```python
from build123d import *

# Parameters (mm, degrees)
BOSS_EXTRUDE1_DEPTH     = 35
SKETCH3_R               = 1.575
CUT_EXTRUDE1_DEPTH      = 10
CUT_EXTRUDE2_DEPTH      = 79.70196948
CUT_EXTRUDE2_DEPTH_BACK = 10
SKETCH5_W               = 10
SKETCH5_H               = 16
FILLET2_R               = 12
FILLET3_R               = 3
FILLET4_R               = 1.5
SKETCH6_W               = 3
SKETCH6_H               = 5.976707935
BOSS_EXTRUDE2_DEPTH     = 15
SKETCH8_R               = 1.125
CUT_EXTRUDE3_DEPTH      = 25
SKETCH10_R              = 3
BOSS_EXTRUDE3_DEPTH     = 3.044394089
SKETCH11_R              = 1.575
CUT_EXTRUDE4_DEPTH      = 7.5


with BuildPart() as part:
    # Sketch2 → Boss-Extrude1 (new body)
    with BuildSketch(Plane.XY):
        Polygon((27, 21), (27, 37), (30, 37), (30, 3), (19, 3), (19, 6), (27, 6), (27, 18), (-27, 18), (-27, 6), (-19, 6), (-19, 3), (-30, 3), (-30, 21), align=None)
    extrude(amount=-BOSS_EXTRUDE1_DEPTH)

    # Sketch3 → Cut-Extrude1 (cut)
    with BuildSketch(Plane(origin=(0, 0, 0), x_dir=(1, 0, 0), z_dir=(0, 1, 0))):
        with Locations(Location((-22.449984171, 16, 0), (0, 0, 90))):
            Circle(SKETCH3_R)
        with Locations(Location((22.550015829, 16, 0), (0, 0, 90))):
            Circle(SKETCH3_R)
    extrude(amount=CUT_EXTRUDE1_DEPTH, mode=Mode.SUBTRACT)

    # Sketch5 → Cut-Extrude2 (cut, two sides: drawn at the far end of the back side and taken through both)
    with BuildSketch(Plane(origin=(30, 0, 0), x_dir=(0, 0, -1), z_dir=(1, 0, 0)).offset(-CUT_EXTRUDE2_DEPTH_BACK)):
        with Locations((5, 29)):
            Rectangle(SKETCH5_W, SKETCH5_H)
    extrude(amount=CUT_EXTRUDE2_DEPTH + CUT_EXTRUDE2_DEPTH_BACK, mode=Mode.SUBTRACT)

    # Fillet2
    fillet2_edges = [part.edges().sort_by_distance(p)[0] for p in [
        (28.5, 37, -10),
        (28.5, 37, -35),
    ]]
    fillet(fillet2_edges, radius=FILLET2_R)

    # Fillet3
    fillet3_edges = [part.edges().sort_by_distance(p)[0] for p in [
        (27, 18, -17.5),
        (-27, 18, -17.5),
        (-30, 21, -17.5),
    ]]
    fillet(fillet3_edges, radius=FILLET3_R)

    # Fillet4
    fillet4_edges = [part.edges().sort_by_distance(p)[0] for p in [
        (19, 6, -17.5),
        (27, 6, -17.5),
        (-27, 6, -17.5),
        (-19, 6, -17.5),
    ]]
    fillet(fillet4_edges, radius=FILLET4_R)

    # Sketch6 → Boss-Extrude2 (add)
    with BuildSketch(Plane(origin=(0, 21, 0), x_dir=(1, 0, 0), z_dir=(0, 1, 0))):
        with Locations((-15.696239988, 32.011646033)):
            Rectangle(SKETCH6_W, SKETCH6_H)
        with Locations((-15.696239988, 2.988353968)):
            Rectangle(SKETCH6_W, SKETCH6_H)
    extrude(amount=BOSS_EXTRUDE2_DEPTH)

    # Sketch8 → Cut-Extrude3 (cut)
    with BuildSketch(Plane(origin=(0, 0, 0), x_dir=(0, 0, -1), z_dir=(1, 0, 0))):
        with Locations(Location((3.473292065, 27.2, 0), (0, 0, 270))):
            Circle(SKETCH8_R)
        with Locations(Location((31.173292065, 27.2, 0), (0, 0, 90))):
            Circle(SKETCH8_R)
    extrude(amount=-CUT_EXTRUDE3_DEPTH, mode=Mode.SUBTRACT)

    # Sketch10 → Boss-Extrude3 (add)
    with BuildSketch(Plane(origin=(30, 0, 0), x_dir=(0, 0, -1), z_dir=(1, 0, 0))):
        with Locations(Location((22.523292065, 27.2, 0), (0, 0, 270))):
            Circle(SKETCH10_R)
    extrude(amount=BOSS_EXTRUDE3_DEPTH)

    # Sketch11 → Cut-Extrude4 (cut, symmetric)
    with BuildSketch(Plane(origin=(30, 0, 0), x_dir=(0, 0, -1), z_dir=(1, 0, 0))):
        with Locations(Location((22.523292065, 27.2, 0), (0, 0, 270))):
            Circle(SKETCH11_R)
    extrude(amount=CUT_EXTRUDE4_DEPTH, both=True, mode=Mode.SUBTRACT)


solid = part.part
```
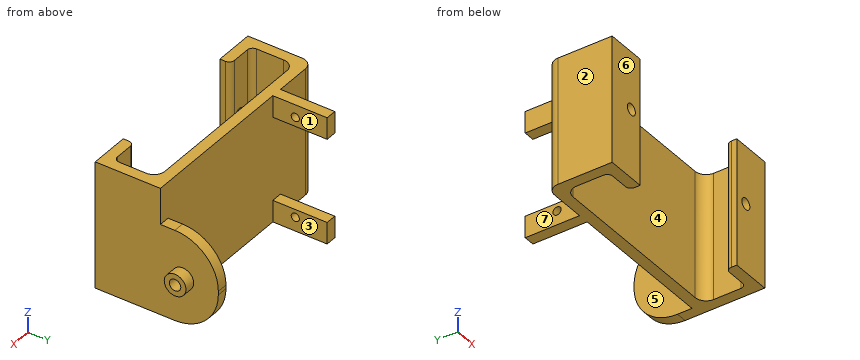
Can you work these out from the model? Positions are in its coordinate system, mm. Face numbers are marked on the shaded views. A direction names the side the tool comes from. Round coordinates to 2 decimals unless told otherwise and drop trailing zeros. Loops run counter-clockwise (first coordinate to the right, second up) from the corner with the lowest first, then second, coordinate; pieces in that order, holes last. Notation, with made-up numbers: M -38,21.5 L 4,21.5 A7 cw 4,32.5 Z; hole C 1.5,83.25 d2. An arc over 180 degrees is marked long. Answer as a JSON object with one key per item and string values. Group by question number.
Q1. We'd pull the mould along X, two halves only. Please class the marked faces 1, 2 and 3: +X half, -X half, draft (parallel to the pull), parting line (faces both ways), or undercut.
Q2. Please list where these lines run through material, in increasing order: L1, parallel to X at y = 4.6, z = -16; L2, parallel to Z at x = -15.75, y = 27.2; L3, parallel to X at y = 4.9, z = -16.
Q3. Imagine slicing it at B-B, the plane y = 23. Please give me the cut outline in (x, z), then the cut area to 3 significant figures.
Q4. Will these pins go through, and if not, where does the flat tip stop? pin 1 (6.5 mm diameter, centred on y = 30, z = -32, fed in from -X); pin 2 (6 mm diameter, centred on x = -0.5, z = -26, fed in from +Y); pin 3 (1.5 mm diameter, centred on x = -15, z = -4, fed in from +Y).
Q5. Imagine slicing it at D-D, the plane y = 27.2. Please give me the cut outline in (x, z), then the cut area to 3 significant figures.
Q6. Imagine slicing it at A-A, the plane y = 14. Please give me the cut outline in (x, z).
Q7. Imagine slicing it at C-C, the plane z = -16. Count the separate pieces of the cut face and the enclosed holes in it, then the cut area to 3 significant figures.
Q8. On a 3-axis mill with a long thin cutter (end or side, diameter ignored), from which of +Z, -Z, +X, -X, +Y, -Y can I reach the whole of each face in a straight line? I mean the marked faces 4, 5, 6 and 7. Say none if no direction works.
Findings:
{
 "1": {"face 1": "+X half", "face 2": "-X half", "face 3": "undercut"},
 "2": {"L1": "x = -30 to -24.02, -20.87 to -19, 19 to 20.98, 24.13 to 30", "L2": "z = -35 to -32.3, -30.05 to -29.02, -5.98 to -4.6, -2.35 to 0", "L3": "x = -30 to -24.02, -20.87 to -19.05, 19.05 to 20.98, 24.13 to 30"},
 "3": {"outline": "M -17.2,-35 L -14.2,-35 L -14.2,-29.02 L -17.2,-29.02 Z; M -17.2,-5.98 L -14.2,-5.98 L -14.2,0 L -17.2,0 Z; M 27,-35 L 30,-35 L 30,-10 L 27,-10 Z", "area": "111 mm2"},
 "4": {"pin 1": "stops at x = -17.2", "pin 2": "stops at y = 21", "pin 3": "stops at y = 36"},
 "5": {"outline": "M -17.2,-35 L -14.2,-35 L -14.2,-32.3 L -17.2,-32.3 Z; M -17.2,-30.05 L -14.2,-30.05 L -14.2,-29.02 L -17.2,-29.02 Z; M -17.2,-5.98 L -14.2,-5.98 L -14.2,-4.6 L -17.2,-4.6 Z; M -17.2,-2.35 L -14.2,-2.35 L -14.2,0 L -17.2,0 Z; M 27,-34.8 L 30,-34.8 L 30,-25.52 L 33.04,-25.52 L 33.04,-24.1 L 27,-24.1 Z; M 27,-20.95 L 33.04,-20.95 L 33.04,-19.52 L 30,-19.52 L 30,-10.2 L 27,-10.2 Z", "area": "95.4 mm2"},
 "6": {"outline": "M -30,-35 L -27,-35 L -27,0 L -30,0 Z; M 27,-35 L 30,-35 L 30,0 L 27,0 Z"},
 "7": {"separate pieces": "3", "enclosed holes": "0", "area": "344 mm2"},
 "8": {"face 4": "+Z, -Z", "face 5": "+Z, -Z, +Y", "face 6": "+Z, -Z, +X, -X, -Y", "face 7": "+Z, -Z, -X, +Y"}
}
